Design review of the part built by this model. Coordinates are the model's own, in mm. Face numbers are marked on the shaded views. A direction names the side the tool comes from. Round coordinates to 2 decimals unless told otherwise and drop trailing zeros. Loops run counter-clockwise (first coordinate to the right, second up) from the corner with the lowest first, then second, coordinate; pieces in that order, holes last. Notation, with made-up numbers: (41.5, -18) - (68.5, -18) arc R9 cw to (68.5, -12) - close; hole circle Ø4 at (23, 89). An arc over 180 degrees is marked (long way). Answer as CSV lines item,"result". Start each with the question number.
(1) Wall thickness on L1, parallel to Z at x = 80, y = 0.5 (3 decimals); L2, parallel to Y at x = -25.5, z = -120; L3, parallel to Y at x = 13, z = 5: over which ranges is each line inside the solid? List them lowest first.
(2) For the marked faces 4, 5, 6, 7 and 8, list the 3-axis set-ups (+Z, -Z, +X, -X, +Y, -Y) from which the entire face can be reached by the end or side of a thin tool; tool diameter is ignored.
(3) Mouldability with a two-part tool opening along Z and no side actions: class the marked faces 1, 2 and 3 as released by +Z, released by -Z, zero draft, split by the parting line, or undercut.
(4) For P1, Ø1, axis at x = 60, y = -24, coming from the +Z side; P2, Ø5, axis at x = -15.5, z = 4, coming from the -Y side; P3, Ø8, axis at y = 45.5, z = -134.5, coming from the -X side, all flat-tipped, find the tip position at first contact; note any pin that passes through.
(5) Consider section B-B (x = 126). Give the boundary of the cut face in (y, z) (3 decimals), and give its area (3 significant figures).
(6) Consider section A-A (z = -30). Give the boundary of the cut face in (x, y), and give its area (3 significant figures).
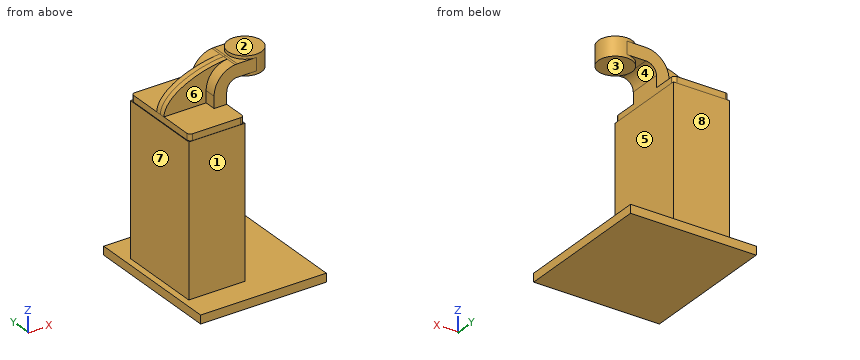
from build123d import *

# Parameters (mm, degrees)
F1_DEPTH  = 63.5
F0_W      = 25.4
F0_H      = 19.05
F2_DEPTH  = 25.4
F3_DEPTH  = 7.9375
F5_R      = 5.08
F6_W      = 84.3743681908
F6_H      = 127.7539134026
F7_DEPTH  = 229.7079414129
F8_W      = 212.6137167215
F8_H      = 12.7539038658
F9_DEPTH  = 51.7011582851
F10_DEPTH = 85.5997037143


# Not quite as in the source:
# - the program builds the solid bodies; features that only make, move or delete a surface that nothing else refers to are left out


with BuildPart() as f1:
    # F0 (on Front) → F1 (new body, symmetric)
    with BuildSketch(Plane.XZ):
        Polygon((22.225, 9.525), (-41.275, 9.525), (-41.275, -9.525), (41.275, -9.525), (41.275, 9.525), align=None)
    extrude(amount=F1_DEPTH, both=True)

    # F0 (on Front) → F2 (join, symmetric)
    with BuildSketch(Plane.XZ):
        with BuildLine():
            Line((22.225, 27.0002), (22.225, 9.525))
            Line((22.225, 9.525), (41.275, 9.525))
            Line((41.275, 9.525), (41.275, 27.0002))
            ThreePointArc((41.275, 27.0002), (45.9246798487, 38.2255201513), (57.15, 42.8752))
            Line((57.15, 42.8752), (60.325, 42.8752))
            Line((60.325, 42.8752), (60.325, 61.9252))
            Line((60.325, 61.9252), (57.15, 61.9252))
            add(Edge.make_bspline(
                [(53.8854342407, 61.7722898912), (54.9842067368, 61.8365871986), (56.0728453275, 61.8876096574), (57.15, 61.9252)],
                knots=[108.5245810491, 108.5245810491, 108.5245810491, 108.5245810491, 111.5045361635, 111.5045361635, 111.5045361635, 111.5045361635], degree=3))
            ThreePointArc((53.8854342407, 61.7722898912), (31.3258777096, 50.5133948686), (22.225, 27.0002))
        make_face()
        with Locations((73.025, 52.4002)):
            Rectangle(F0_W, F0_H)
    extrude(amount=F2_DEPTH, both=True)

    # F0 (on Front) → F3 (join, symmetric)
    with BuildSketch(Plane.XZ):
        with BuildLine():
            add(Edge.make_bspline(
                [(-41.275, 9.525), (-39.5856284224, 39.4828766469), (13.870125209, 59.4306981306), (53.8854342407, 61.7722898912)],
                knots=[0, 0, 0, 0, 108.5245810491, 108.5245810491, 108.5245810491, 108.5245810491], degree=3))
            Line((-41.275, 9.525), (22.225, 9.525))
            Line((22.225, 9.525), (22.225, 27.0002))
            ThreePointArc((22.225, 27.0002), (31.3258777096, 50.5133948686), (53.8854342407, 61.7722898912))
        make_face()
    extrude(amount=F3_DEPTH, both=True)

    # F0 (on Front) → F4 (revolve)
    with BuildSketch(Plane.XZ):
        Polygon((85.725, 66.675), (85.725, 61.9252), (85.725, 42.8752), (85.725, 38.1), (111.125, 38.1), (111.125, 66.675), align=None)
    revolve(axis=Axis((85.725, 0, 52.3875), (0, 0, 1)))

    # F5
    f5_edges = [f1.edges().sort_by_distance(p)[0] for p in [
        (41.275, -63.5, 0),
        (-41.275, -63.5, 0),
        (41.275, 63.5, 0),
        (-41.275, 63.5, 0),
    ]]
    fillet(f5_edges, radius=F5_R)

    # F6 (on Top) → F7 (join)
    with BuildSketch(Plane.XY):
        Rectangle(F6_W, F6_H)
    extrude(amount=-F7_DEPTH)

    # F8 (on Right) → F9 (join, symmetric)
    with BuildSketch(Plane.YZ):
        with Locations((2.6118680835, -230.9240400791)):
            Rectangle(F8_W, F8_H)
    extrude(amount=F9_DEPTH, both=True)

    # F10 (add): a face of the model
    f10_faces = [f1.faces().sort_by_distance(p)[0] for p in [
        (51.7011582851, 2.6118680835, -230.9240400791),
    ]]
    extrude(f10_faces, amount=F10_DEPTH)


solid = f1.part
Determined:
1,L1,"z = -237.301 to -224.547, 38.1 to 66.675"
1,L2,"y = -63.88 to 63.88"
1,L3,"y = -63.5 to 63.5"
2,face 4,"+Y, -Y"
2,face 5,"+X, +Y, -Y"
2,face 6,"+Z, -X, -Y"
2,face 7,"+Z, -X, +Y, -Y"
2,face 8,"+Z, +X, -X, +Y"
3,face 1,"zero draft"
3,face 2,"released by +Z"
3,face 3,"undercut"
4,P1,"stops at z = 61.93"
4,P2,"stops at y = -63.5"
4,P3,"stops at x = -42.19"
5,outline,"(-103.695, -237.301) - (108.919, -237.301) - (108.919, -224.547) - (-103.695, -224.547) - close"
5,area,"2,710 mm^2"
6,outline,"(-42.19, -63.88) - (42.19, -63.88) - (42.19, 63.88) - (-42.19, 63.88) - close"
6,area,"10,800 mm^2"
